Geometry: final body of the model. Coordinates: model frame, mm. A direction names the side the tool comes from. Give positions to 0.01 mm unless a question says otherwise; leave off trailing zeros. Loops run counter-clockwise (first coordinate to the right, second up) from the corner with the lowest first, then second, coordinate; pieces in that order, holes last. Notation, with made-up numbers: (66.5, 64) - (106.5, 64) arc R6 cw to (106.5, 75) - close; hole circle Ø6 at (86.25, -11.5). An arc over 180 degrees is marked (long way). Use one line per item in the form item = value.
Autodesk Inventor part; units mm, degrees
ref_plane "YZ Plane" through (0, 0, 0) normal (1, 0, 0) x (0, 1, 0)
ref_plane "XZ Plane" through (0, 0, 0) normal (0, 1, 0) x (-1, 0, 0)
ref_plane "XY Plane" through (0, 0, 0) normal (0, 0, 1) x (1, 0, 0)
sketch "스케치1" plane through (0, 0, 0) normal (0, 1, 0) x (-1, 0, 0)
  line L0 (0, 0) -> (-19, 0)
  line L1 (-19, 0) -> (-19, -17)
  line L2 (-19, -17) -> (0, -17)
  line L3 (0, -17) -> (0, 0)
  dimension "d0" = 17
  dimension "d1" = 19
extrude "돌출1" add sketch "스케치1" along normal blind 7.6
sketch "스케치2" plane through (0, 0, 0) normal (0, 0, 1) x (1, 0, 0)
  circle A0 centre (9.5, 3.8) radius 2.5
  line L0 (0, 7.6) -> (19, 7.6)
  line L1 (19, 0) -> (19, 7.6)
  point P0 (0, 0)
  point P1 (9.5, 7.6)
  point P2 (19, 3.8)
  dimension "d4" = 5
extrude "돌출2" cut sketch "스케치2" against normal blind 10
properties part number "loadcell"
(1) Cut plane B-B (y = 3.8). Return the cut outline in (x, z).
Solution:
outline = (0, -17) - (19, -17) - (19, 0) - (12, 0) - (12, -10) - (7, -10) - (7, 0) - (0, 0) - close
(2) Pin query (flat end, axial travel): P1, Ø1.5, axis at x = 10, y = 4.5, coming from the +Z side; P2, Ø1.5, axis at y = 2.5, z = -5, coming from the -X side. Return the tip coordinate at first contact, or that it passes through.
Solution:
P1 = -10
P2 = 0
(3) Pull-direction query (Y, two-part tool) for faces 1 (the face through (8.96, 1.36, -4.93)), 2 (the face through (10, 0, -8)), 3 (the face through (10, 4, -17)); classes: released by +Y, released by -Y, zero draft, split by the parting line, or undercut.
Solution:
face_1 = undercut
face_2 = released by -Y
face_3 = zero draft
(4) Access query for faces 4 (the face through (9, 1, 0)), 5 (the face through (9, 4, -10)). Directions: +Z, -Z, +X, -X, +Y, -Y. A direction counts if a zero-diameter tool reaches every point of the face in a straight line with its end or side. Return the directions, or none.
Solution:
face_4 = +Z, +X, -X, +Y, -Y
face_5 = +Z
(5) Cut plane A-A (z = -6.25). Return the cut outline in (x, y).
Solution:
outline = (0, 0) - (19, 0) - (19, 7.6) - (0, 7.6) - close; hole circle Ø5 at (9.5, 3.8)
(6) Cut plane C-C (x = 9.5). Return the cut outline in (y, z), plus the area to 3 significant figures.
Solution:
outline = (0, -17) - (7.6, -17) - (7.6, 0) - (6.3, 0) - (6.3, -10) - (1.3, -10) - (1.3, 0) - (0, 0) - close
area = 79.2 mm2
(7) Material intervals for L1, parallel to Y at x = 9.5, z = -7; L2, parallel to Z at x = 10.75, y = 4; L3, parallel to X at y = 3, z = -1.25, sorted ascending. Write a range as from..to.
Solution:
L1 = 0..1.3, 6.3..7.6
L2 = -17..-10
L3 = 0..7.13, 11.87..19
